Design review of the part built by this model. Coordinates are the model's own, in mm. A direction names the side the tool comes from. Give positions to 0.01 mm unless a question says otherwise; leave off trailing zeros. Write each loop counter-clockwise with the first axis right and the second up, starting at its lowest first coordinate (ties: lowest second). Pieces come first, ordered by that corner, then holes. Notation, with made-up numbers: M 38.5,44 L 86.5,44 A11 cw 86.5,55 Z; hole C 59.5,19.25 d10. An arc over 180 degrees is marked long. Use a Markdown table: item, result. Add a question column.
```python
from build123d import *

# Parameters (mm, degrees)
EXTRUDE_1_DEPTH     = 7
SKETCH_2_R          = 10.5
CUT_EXTRUDE_1_DEPTH = 3.5
SKETCH_3_R          = 5
CUT_EXTRUDE_2_DEPTH = 69.914802474
EXTRUDE_START       = 5.2
EXTRUDE_2_DEPTH     = 5.2
CUT_EXTRUDE_START   = -10.220454921
CUT_EXTRUDE_3_DEPTH = 45.240565609
CHAMFER_1_SIZE      = 0.5
CHAMFER_2_SIZE      = 0.3
CHAMFER_3_SIZE      = 0.3
CHAMFER_3_SIZE_2    = 0.254518099
CHAMFER_3_SIZE_3    = 0.383899621
CHAMFER_3_SIZE_4    = 0.356772393
CHAMFER_3_SIZE_5    = 0.263835418


with BuildPart() as part:
    # 草图1 → 凸台-拉伸1 (new body)
    with BuildSketch(Plane.XY):
        with BuildLine():
            Line((0.9, -11.966202405), (60.5625, -7.478876503))
            ThreePointArc((60.5625, -7.478876503), (67.5, 0), (60.5625, 7.478876503))
            Line((60.5625, 7.478876503), (0.9, 11.966202405))
            ThreePointArc((0.9, 11.966202405), (-12, 0), (0.9, -11.966202405))
        make_face()
    extrude(amount=EXTRUDE_1_DEPTH)

    # 草图2 → 切除-拉伸1 (cut)
    with BuildSketch(Plane.XY.offset(7)):
        Circle(SKETCH_2_R)
    extrude(amount=-CUT_EXTRUDE_1_DEPTH, mode=Mode.SUBTRACT)

    # 草图3 → 切除-拉伸2 (cut, through all)
    with BuildSketch(Plane(origin=(0, 0, 0), x_dir=(-1, 0, 0), z_dir=(0, 0, -1))):
        Circle(SKETCH_3_R)
    extrude(amount=-CUT_EXTRUDE_2_DEPTH, mode=Mode.SUBTRACT)

    # 草图4 → 凸台-拉伸2 (add)
    with BuildSketch(Plane(origin=(0, 0, 0), x_dir=(-1, 0, 0), z_dir=(0, 0, -1)).offset(EXTRUDE_START)):
        with BuildLine():
            Line((-24.349176843, -10.202546866), (-34.487976367, 9.439989183))
            Line((-34.487976367, 9.439989183), (-60.5625, 7.478876503))
            ThreePointArc((-60.5625, 7.478876503), (-67.5, 0), (-60.5625, -7.478876503))
            Line((-60.5625, -7.478876503), (-24.349176843, -10.202546866))
        make_face()
    extrude(amount=-EXTRUDE_2_DEPTH)

    # 切除-拉伸3: read off the stored shape, not the designer's step
    # 切除-拉伸3 outline → 切除-拉伸3 (cut)
    with BuildSketch(Plane(origin=(0, 0, 0), x_dir=(0.8886074479712769, -0.45866851146549686, 0), z_dir=(0.45866851146549686, 0.8886074479712767, 0)).offset(CUT_EXTRUDE_START)):
        Polygon((26.316446878, 5.2), (26.316446878, 0), (39.011877148, 5.2), align=None)
        Polygon((62, -7), (62, -1.8), (40.108675427, -1.8), (27.413245157, -7), align=None)
    extrude(amount=CUT_EXTRUDE_3_DEPTH, mode=Mode.SUBTRACT)

    # 草图6 → 切除-旋转1 (revolve, cut)
    with BuildSketch(Plane(origin=(0, 0, 0), x_dir=(1, 0, 0), z_dir=(0, 1, 0))):
        Polygon((60, 5.2), (58, 5.2), (58, 1.7), (56, 1.7), (56, -1.8), (60, -1.8), align=None)
    revolve(axis=Axis((60, 0, -13.45), (0, 0, 1)), mode=Mode.SUBTRACT)

    # 倒角1
    chamfer_1_edges = [part.edges().sort_by_distance(p)[0] for p in [
        (-10.5, 0, 7),
    ]]
    chamfer(chamfer_1_edges, length=CHAMFER_1_SIZE)

    # 倒角2
    chamfer_2_edges = [part.edges().sort_by_distance(p)[0] for p in [
        (62, 0, -5.2),
    ]]
    chamfer(chamfer_2_edges, length=CHAMFER_2_SIZE)

    # 倒角3
    # the kernel refuses this chamfer: 0.383899621, 0.356772393, 0.3, 0.263835418, 0.254518099 mm, written as the material it takes off along each edge
    with BuildSketch(Plane(origin=(60.5625, -7.478876503, -5.2), x_dir=(-0.07499999999999998, 0.9971835337589565, 0), z_dir=(-0.9971835337589565, -0.07499999999999998, 0))) as chamfer_3_piece_1:
        Polygon((CHAMFER_3_SIZE, 0), (0, -CHAMFER_3_SIZE), (0, 0), align=None)
    extrude(amount=22.721254915, mode=Mode.SUBTRACT)
    with BuildSketch(Plane(origin=(60, 0, -5.2), x_dir=(0.07499999999999998, 0.9971835337589565, 0), z_dir=(-0.9971835337589565, 0.07499999999999998, 0))) as chamfer_3_piece_2:
        Polygon((7.5 - CHAMFER_3_SIZE, 0), (7.5, -CHAMFER_3_SIZE), (7.5, 0), align=None)
    revolve(axis=Axis((60, 0, -5.2), (0, 0, -1)), revolution_arc=171.397555391, mode=Mode.SUBTRACT)
    with BuildSketch(Plane(origin=(46.933080248, 8.503970126, -5.2), x_dir=(-0.07499999999999997, -0.9971835337589565, 0), z_dir=(0.9971835337589565, -0.07499999999999997, 0))) as chamfer_3_piece_3:
        Polygon((CHAMFER_3_SIZE, 0), (0, -CHAMFER_3_SIZE), (0, 0), align=None)
    extrude(amount=13.667914973, mode=Mode.SUBTRACT)
    # the kernel refuses this chamfer: 0.383899621, 0.356772393, 0.3, 0.263835418, 0.254518099 mm, written as the material it takes off along each edge
    with BuildSketch(Plane(origin=(0.9, -11.966202405, 0), x_dir=(-0.07499999999999997, 0.9971835337589565, 0), z_dir=(0.9971835337589566, 0.07499999999999997, 0))) as chamfer_3_2_piece_1_section:
        Polygon((CHAMFER_3_SIZE, 0), (0, CHAMFER_3_SIZE), (0, 0), align=None)
    chamfer_3_2_piece_1 = extrude(amount=24.286912089, mode=Mode.PRIVATE)
    chamfer_3_2_piece_1 = split(chamfer_3_2_piece_1, bisect_by=Plane(origin=(3.45685625, -13.285963401, 7.024904811), z_dir=(-0.33681186979171107, 0.17385066860959783, -0.9253830068633244)), keep=Keep.TOP, mode=Mode.PRIVATE)
    add(chamfer_3_2_piece_1, mode=Mode.SUBTRACT)
    with BuildSketch(Plane(origin=(35.257308346, 9.382126316, 0), x_dir=(0, 0, 1), z_dir=(-0.9971835337589566, 0.075, 0))) as chamfer_3_2_piece_2_section:
        Polygon((CHAMFER_3_SIZE, 0), (0, -CHAMFER_3_SIZE), (0, 0), align=None)
    chamfer_3_2_piece_2 = extrude(amount=34.454347854, mode=Mode.PRIVATE)
    chamfer_3_2_piece_2 = split(chamfer_3_2_piece_2, bisect_by=Plane(origin=(35.166645448, 9.428923377, -0.249094265), z_dir=(-0.33681186979171107, 0.17385066860959783, -0.9253830068633244)), keep=Keep.TOP, mode=Mode.PRIVATE)
    add(chamfer_3_2_piece_2, mode=Mode.SUBTRACT)
    with BuildSketch(Plane(origin=(0, 0, 0), x_dir=(0.07500000000000011, 0.9971835337589566, 0), z_dir=(0.9971835337589566, -0.07500000000000011, 0))) as chamfer_3_2_piece_3:
        Polygon((12 - CHAMFER_3_SIZE, 0), (12, CHAMFER_3_SIZE), (12, 0), align=None)
    revolve(axis=Axis((0, 0, 0), (0, 0, 1)), revolution_arc=188.602444609, mode=Mode.SUBTRACT)
    # the kernel refuses this chamfer: 0.383899621, 0.356772393, 0.3, 0.263835418, 0.254518099 mm, written as the material it takes off along each edge
    with BuildSketch(Plane(origin=(39.590447843, -9.056222958, -5.332010389), x_dir=(0.3284593891924205, 0.024704032262311923, 0.9441949695064703), z_dir=(-0.9415356762498924, -0.07081462271298539, 0.3293870968308798))) as chamfer_3_3_piece_1_section:
        Polygon((CHAMFER_3_SIZE_2 * 0.999999998644, 0), (CHAMFER_3_SIZE * 0.198621914305, CHAMFER_3_SIZE * 0.980076188446), (0, 0), align=None)
    chamfer_3_3_piece_1 = extrude(amount=17.869959702, mode=Mode.PRIVATE)
    chamfer_3_3_piece_1 = split(chamfer_3_3_piece_1, bisect_by=Plane(origin=(39.379247454, -6.248148947, -2.516005194), z_dir=(0.05303300858899107, -0.7051152388085232, -0.7071067811865471)), keep=Keep.TOP, mode=Mode.PRIVATE)
    add(chamfer_3_3_piece_1, mode=Mode.SUBTRACT)
    # the kernel refuses this chamfer: 0.383899621, 0.356772393, 0.3, 0.263835418, 0.254518099 mm, written as the material it takes off along each edge
    with BuildSketch(Plane(origin=(39.727912607, -9.045883981, 1.8), x_dir=(-0.07499999999999996, 0.9971835337589565, 0), z_dir=(0.9971835337589566, 0.07499999999999997, 0))) as chamfer_3_4_piece_1_section:
        Polygon((CHAMFER_3_SIZE, 0), (0, -CHAMFER_3_SIZE), (0, 0), align=None)
    chamfer_3_4_piece_1 = extrude(amount=20.893433042, mode=Mode.PRIVATE)
    chamfer_3_4_piece_1 = split(chamfer_3_4_piece_1, bisect_by=Plane(origin=(39.811799189, -9.089183341, 2.030476488), z_dir=(0.33681186979171107, -0.17385066860959783, 0.9253830068633244)), keep=Keep.TOP, mode=Mode.PRIVATE)
    add(chamfer_3_4_piece_1, mode=Mode.SUBTRACT)
    with BuildSketch(Plane(origin=(60, 0, 1.8), x_dir=(0.075, 0.9971835337589565, 0), z_dir=(-0.9971835337589565, 0.075, 0))) as chamfer_3_4_piece_2:
        Polygon((7.5 - CHAMFER_3_SIZE, 0), (7.5, CHAMFER_3_SIZE), (7.5, 0), align=None)
    revolve(axis=Axis((60, 0, 1.8), (0, 0, -1)), revolution_arc=171.397555391, mode=Mode.SUBTRACT)
    with BuildSketch(Plane(origin=(60.5625, 7.478876503, 1.8), x_dir=(-0.07499999999999998, -0.9971835337589565, 0), z_dir=(-0.9971835337589566, 0.075, 0))) as chamfer_3_4_piece_3_section:
        Polygon((CHAMFER_3_SIZE, 0), (0, -CHAMFER_3_SIZE), (0, 0), align=None)
    chamfer_3_4_piece_3 = extrude(amount=11.936343353, mode=Mode.PRIVATE)
    chamfer_3_4_piece_3 = split(chamfer_3_4_piece_3, bisect_by=Plane(origin=(59.250471243, 8.156100488, -1.804769384), z_dir=(0.33681186979171107, -0.17385066860959783, 0.9253830068633244)), keep=Keep.TOP, mode=Mode.PRIVATE)
    add(chamfer_3_4_piece_3, mode=Mode.SUBTRACT)
    # the kernel refuses this chamfer: 0.383899621, 0.356772393, 0.3, 0.263835418, 0.254518099 mm, written as the material it takes off along each edge
    with BuildSketch(Plane(origin=(42.288756392, -8.85327823, 1.173257023), x_dir=(-0.3284593891924201, -0.02470403226231695, -0.9441949695064704), z_dir=(-0.9415356762498924, -0.07081462271298539, 0.3293870968308797))) as chamfer_3_5_piece_1_section:
        Polygon((CHAMFER_3_SIZE_3 * 1.0000000011, 0), (-CHAMFER_3_SIZE * 0.198621914305, -CHAMFER_3_SIZE * 0.980076188446), (0, 0), align=None)
    chamfer_3_5_piece_1 = extrude(amount=19.376005008, mode=Mode.PRIVATE)
    chamfer_3_5_piece_1 = split(chamfer_3_5_piece_1, bisect_by=Plane(origin=(42.301009253, -9.016189588, 1.336628512), z_dir=(0.053033008588990585, -0.7051152388085168, 0.7071067811865535)), keep=Keep.TOP, mode=Mode.PRIVATE)
    add(chamfer_3_5_piece_1, mode=Mode.SUBTRACT)
    # the kernel refuses this chamfer: 0.383899621, 0.356772393, 0.3, 0.263835418, 0.254518099 mm, written as the material it takes off along each edge
    with BuildSketch(Plane(origin=(0.9, -11.966202405, 7), x_dir=(-0.07499999999999997, 0.9971835337589565, 0), z_dir=(0.9971835337589566, 0.07499999999999997, 0))) as chamfer_3_6_piece_1:
        Polygon((CHAMFER_3_SIZE, 0), (0, -CHAMFER_3_SIZE), (0, 0), align=None)
    extrude(amount=25.952193485, mode=Mode.SUBTRACT)
    with BuildSketch(Plane(origin=(36.984003052, 9.252258445, 7), x_dir=(-0.075, -0.9971835337589565, 0), z_dir=(-0.9971835337589566, 0.075, 0))) as chamfer_3_6_piece_2:
        Polygon((CHAMFER_3_SIZE, 0), (0, -CHAMFER_3_SIZE), (0, 0), align=None)
    extrude(amount=36.185919473, mode=Mode.SUBTRACT)
    with BuildSketch(Plane(origin=(0, 0, 7), x_dir=(0.07500000000000011, 0.9971835337589566, 0), z_dir=(0.9971835337589566, -0.07500000000000011, 0))) as chamfer_3_6_piece_3:
        Polygon((12 - CHAMFER_3_SIZE, 0), (12, -CHAMFER_3_SIZE), (12, 0), align=None)
    revolve(axis=Axis((0, 0, 7), (0, 0, 1)), revolution_arc=188.602444609, mode=Mode.SUBTRACT)
    # the kernel refuses this chamfer: 0.383899621, 0.356772393, 0.3, 0.263835418, 0.254518099 mm, written as the material it takes off along each edge
    with BuildSketch(Plane(origin=(32.83531163, 9.564289125, 0.624872862), x_dir=(-0.12627439013591127, -0.9822683171715932, -0.13857752875805598), z_dir=(0.9330662049196804, -0.07017761826168661, -0.3527925156971192))) as chamfer_3_7_piece_1_section:
        Polygon((CHAMFER_3_SIZE, 0), (-CHAMFER_3_SIZE_4 * 0.148100133729, -CHAMFER_3_SIZE_4 * 0.988972370164), (0, 0), align=None)
    chamfer_3_7_piece_1 = extrude(amount=17.22586636, mode=Mode.PRIVATE)
    chamfer_3_7_piece_1 = split(chamfer_3_7_piece_1, bisect_by=Plane(origin=(32.847494362, 9.72626806, 0.462436431), z_dir=(0.05303300858899109, 0.7051152388085231, -0.7071067811865475)), keep=Keep.TOP, mode=Mode.PRIVATE)
    add(chamfer_3_7_piece_1, mode=Mode.SUBTRACT)
    # the kernel refuses this chamfer: 0.383899621, 0.356772393, 0.3, 0.263835418, 0.254518099 mm, written as the material it takes off along each edge
    with BuildSketch(Plane(origin=(35.245808416, 9.382991247, 7.162707961), x_dir=(-0.351798887486564, 0.026459438677302174, -0.935701576822492), z_dir=(0.9330662049196804, -0.07017761826168642, -0.35279251569711917))) as chamfer_3_8_piece_1_section:
        Polygon((CHAMFER_3_SIZE_5 * 1.00000000141, 0), (CHAMFER_3_SIZE * 0.148100133836, -CHAMFER_3_SIZE * 0.988972370877), (0, 0), align=None)
    chamfer_3_8_piece_1 = extrude(amount=16.82260493, mode=Mode.PRIVATE)
    chamfer_3_8_piece_1 = split(chamfer_3_8_piece_1, bisect_by=Plane(origin=(35.033456868, 6.559611679, 4.33135398), z_dir=(0.05303300858899218, 0.7051152388085377, 0.7071067811865327)), keep=Keep.TOP, mode=Mode.PRIVATE)
    add(chamfer_3_8_piece_1, mode=Mode.SUBTRACT)


solid = part.part
```
(1) Wall thickness on L1, parallel to Y at x = 0, z = 1.75; L2, parallel to Z at x = 51, y = 7.75; L3, parallel to Z at x = 19.5, y = -8.5: over which ranges is each line inside the solid? List them lowest first.
(2) Add section B-B on y = 0. Give the number of separate pieces and of enclosed holes in the cut face, then the cut area to 3 significant figures.
(3) Add section D-D on x = 55. Give the boundary of the cut face in (y, z), then the cut area to 3 significant figures.
(4) Add section A-A on x = 0. Give the boundary of the cut face in (y, z).
(5) The part is to be moulded in two halves that separate along X. For faces 1 (the flat face through (11, 0, 0)), 2 (the flat face through (36.126, -1.017, -2.561)), 3 (the cylindrical face through (56.185, -1.201, 0.075)), say which applies: released by +X, released by -X, zero draft, split by the parting line, or undercut.
(6) Machinability: for faces 4 (the conical face through (67.32, 0.15, -5.08)), 5 (the cylindrical face through (10, 3.2, 5)), 6 (the flat face through (53, -2, 1.8)), which of the approach directions +Z, -Z, +X, -X, +Y, -Y give a long, thin tool a straight path to every point of the face, cutting with its end or side? Answer none if there is none.
(7) For pin 1 (8 mm diameter, centred on x = 51.5, y = -5, fed in from +Z); pin 2 (5 mm diameter, centred on x = 14, z = 2.5, fed in from -Y); pin 3 (2 mm diameter, centred on x = 44.5, y = 7, fed in from -Z), all flat-tipped, find the tip position at first contact; note any pin that passes through.
(8) Add section C-C on z = -2.75. Give the boundary of the cut face in (x, y), then the cut area to 3 significant figures.
From the geometry:
| question | item | result |
|---|---|---|
| 1 | L1 | y = -12 to -5, 5 to 12 |
| 1 | L2 | z = -5.2 to 1.8 |
| 1 | L3 | z = 0 to 7 |
| 2 | separate pieces | 3 |
| 2 | enclosed holes | 0 |
| 2 | area | 412 mm^2 |
| 3 | outline | M -7.9,-4.9 L -7.6,-5.2 L 7.6,-5.2 L 7.9,-4.9 L 7.9,1.5 L 7.6,1.8 L -7.6,1.8 L -7.9,1.5 Z |
| 3 | area | 110 mm^2 |
| 4 | outline | M -12,0.3 L -11.7,0 L -5,0 L -5,3.5 L -10.5,3.5 L -10.5,6.5 L -11,7 L -11.7,7 L -12,6.7 Z; M 5,0 L 11.7,0 L 12,0.3 L 12,6.7 L 11.7,7 L 11,7 L 10.5,6.5 L 10.5,3.5 L 5,3.5 Z |
| 5 | face 1 | zero draft |
| 5 | face 2 | released by -X |
| 5 | face 3 | undercut |
| 6 | face 4 | -Z, +X |
| 6 | face 5 | +Z |
| 6 | face 6 | +Z, +X, -Y |
| 7 | pin 1 | stops at z = 1.8 |
| 7 | pin 2 | stops at y = -11.17 |
| 7 | pin 3 | stops at z = -4.51 |
| 8 | outline | M 32.37,-9.3 L 32.98,-9.55 L 60.56,-7.48 A7.5 ccw 60.56,7.48 L 42.77,8.82 L 41.61,8.61 Z; hole C 60,0 d4 |
| 8 | area | 460 mm^2 |
